Geometry: final body of the model. Coordinates: model frame, mm. Face numbers are marked on the shaded views. A direction names the side the tool comes from. Give positions to 0.01 mm unless a question says otherwise; leave off trailing zeros. Loops run counter-clockwise (first coordinate to the right, second up) from the corner with the lowest first, then second, coordinate; pieces in that order, holes last. Notation, with made-up numbers: (56.5, -1) -> (66.5, -1) arc R23 ccw to (66.5, 15) -> close; hole circle Ø10 at (53.5, 73). An arc over 180 degrees is marked (long way). Answer in a Markdown table with one row per item. Add a question column.
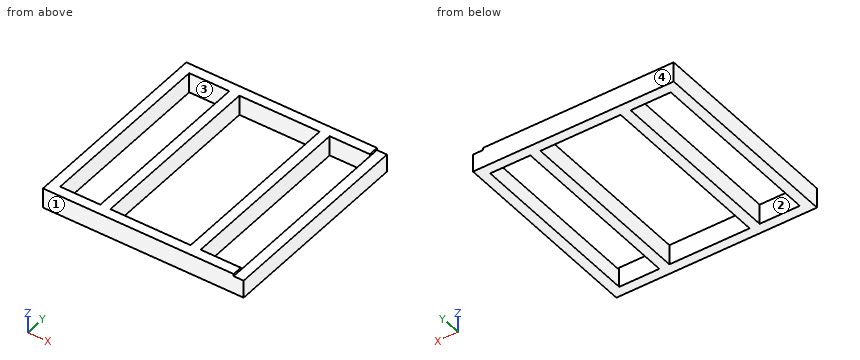
from build123d import *

# Parameters (mm, degrees)
F0_W        = 101.6
F0_H        = 457.1899072886
F0_W_2      = 203.2
F0_H_2      = 25.4
F1_DEPTH    = 50.8
F2_T        = 45.085
F2_T3_DEPTH = 140.97


# Not quite as in the source:
# - a shell that OpenCascade refuses in one call is made with other operations: the cavity is built on its own and cut out


with BuildPart() as f1:
    # F0 (on Top) → F1 (new body)
    with BuildSketch(Plane.XY):
        Polygon((-228.6, 213.5899730921), (-254, 213.5899730921), (-254, 188.1798803806), (-254, -213.5899730921), (-254, -294.4100269079), (-228.6, -294.4100269079), (-127, -294.4100269079), (-101.6, -294.4100269079), (-101.6, -269.0100269079), (-101.6, 188.1798803806), (-101.6, 188.1899730921), (101.6, 188.1899730921), (101.6, -269.0100269079), (101.6, -294.4100269079), (254, -294.4100269079), (254, -269.0100269079), (254, 213.5899730921), (101.6, 213.5899730921), (-101.6, 213.5899730921), (-127, 213.5899730921), align=None)
        with Locations((-177.8, -40.4150732636)):
            Rectangle(F0_W, F0_H, mode=Mode.SUBTRACT)
        with Locations((177.8, -40.4150732636)):
            Rectangle(F0_W, F0_H, mode=Mode.SUBTRACT)
        with Locations((0, -281.7100269079)):
            Rectangle(F0_W_2, F0_H_2)
    extrude(amount=F1_DEPTH)

    # F2: shell of thickness 45.085, made by hand


with BuildPart() as f2_core1:
    # F2_t2: copy of F1
    add(f1.part)

    # the walls: a layer under each face that stays
    f2_faces = [f2_core1.faces().sort_by_distance(p)[0] for p in [
        (-101.6, -40.4100269079, 25.4),
        (0, 188.1899730921, 25.4),
        (0, -269.0100269079, 25.4),
        (-228.6, -40.4150732636, 25.4),
        (-177.8, 188.1798803806, 25.4),
        (-177.8, -269.0100269079, 25.4),
        (177.8, 188.1798803806, 25.4),
        (177.8, -269.0100269079, 25.4),
        (127, -40.4150732636, 25.4),
        (-237.0666666667, -277.4766935746, 0),
    ]]
    thicken(f2_faces, amount=-F2_T, mode=Mode.SUBTRACT)

    # F2_s4 → F2_t3 (cut)
    with BuildSketch(Plane.XY.offset(-45.085)):
        Polygon((-101.14915, -268.5591769079), (-146.685, -269.0100269079), (-146.685, -314.0950269079), (-101.6, -314.0950269079), align=None)
        Polygon((-101.14915, 187.7391230921), (-146.685, 188.1899730921), (-146.685, 233.2749730921), (-101.6, 233.2749730921), align=None)
        Polygon((-228.14915, -268.5591769079), (-273.685, -269.0100269079), (-273.685, -314.0950269079), (-228.6, -314.0950269079), align=None)
        Polygon((-228.14915, 187.7290303806), (-273.685, 188.1798803806), (-273.685, 233.2648803806), (-228.6, 233.2648803806), align=None)
        Polygon((127.45085, 187.7290303806), (127, 233.2648803806), (81.915, 233.2648803806), (81.915, 188.1798803806), align=None)
        Polygon((127.45085, -268.5591769079), (127, -314.0950269079), (81.915, -314.0950269079), (81.915, -269.0100269079), align=None)
    extrude(amount=F2_T3_DEPTH, mode=Mode.SUBTRACT)


with BuildPart() as f1_1:
    add(f1.part)

    # what is left inside the walls is the cavity
    f2_cavity = [f2_core1.part.solids().sort_by_distance(p)[0] for p in [
        (241.3, -125.076694, 45.53585),
    ]]
    add(f2_cavity, mode=Mode.SUBTRACT)


solid = f1_1.part
(1) Pin query (flat end, axial travel): pin 1 Ø1.7 at (y, z) = (197.5, 49) entering from +X; pin 2 Ø5 at (x, y) = (115.5, 14) entering from -Z; pin 3 Ø12.5 at (x, y) = (236.5, -23) entering from +Z (3 decimals). Return the tip coordinate at first contact, or that it passes through.
(2) Cut plane C-C on z = 20.5. Return the cut outline in (x, y).
(3) Reachability of the marked faces 3 and 4 from +Z, -Z, +X, -X, +Y, -Y: full face, straight path, thin tool, end or side. Return the list, or none.
(4) Draft query along X for the marked faces 1 and 2. Return one class per face: +X half, -X half, draft (parallel to the pull), parting line (faces both ways), or undercut.
(5) Cut plane B-B on y = -1.5. Return the cut outline in (x, z) (3 decimals), then the cut area to 3 significant figures.
(6) Material intervals for line 1 along X through (y, z) = (33, 44); line 2 along Y through (x, z) = (-155, 35), sorted ascending. Write a range as from..to.
(7) Cut plane A-A on x = 209. Return the cut outline in (y, z).
(8) Cut plane D-D on x = 62.5. Return the cut outline in (y, z).
Answer list:
| question | item | result |
|---|---|---|
| 1 | pin 1 | stops at x = 228.6 |
| 1 | pin 2 | stops at z = 0 |
| 1 | pin 3 | stops at z = 45.085 |
| 2 | outline | (-254, -294.41) -> (254, -294.41) -> (254, 213.59) -> (-254, 213.59) -> close; hole (-228.6, -269.01) -> (-127, -269.01) -> (-127, 188.18) -> (-228.6, 188.18) -> close; hole (-101.6, -269.01) -> (101.6, -269.01) -> (101.6, 188.19) -> (-101.6, 188.19) -> close; hole (127, -269.01) -> (228.6, -269.01) -> (228.6, 188.18) -> (127, 188.18) -> close |
| 3 | face 3 | +Z, -Z |
| 3 | face 4 | +Z, -Z, +X, -X, +Y |
| 4 | face 1 | draft |
| 4 | face 2 | undercut |
| 5 | outline | (-254, 0) -> (-228.6, 0) -> (-228.6, 50.8) -> (-254, 50.8) -> close; (-127, 0) -> (-101.6, 0) -> (-101.6, 50.8) -> (-127, 50.8) -> close; (101.6, 0) -> (127, 0) -> (127, 50.8) -> (101.6, 50.8) -> close; (228.6, 0) -> (254, 0) -> (254, 45.085) -> (228.6, 45.085) -> close |
| 5 | area | 5,020 mm² |
| 6 | line 1 | x = -254..-228.6, -127..-101.6, 101.6..127, 228.6..254 |
| 6 | line 2 | y = -294.41..-269.01, 188.18..213.59 |
| 7 | outline | (-294.41, 0) -> (-269.01, 0) -> (-269.01, 50.8) -> (-294.41, 50.8) -> close; (188.18, 0) -> (213.59, 0) -> (213.59, 50.8) -> (188.18, 50.8) -> close |
| 8 | outline | (-294.41, 0) -> (-269.01, 0) -> (-269.01, 50.8) -> (-294.41, 50.8) -> close; (188.19, 0) -> (213.59, 0) -> (213.59, 50.8) -> (188.19, 50.8) -> close |
